Read the model definition and answer for the solid it produces. Units are mm, in the model's axes. A direction names the side the tool comes from. Give positions to 0.01 mm unless a question says otherwise; leave off trailing zeros. Order: outer loops, then holes, each group sorted by start corner. A loop starts at its lowest first (then second) coordinate and runs counter-clockwise, first axis right, second up.
Item 1: Given pin 1 Ø1.5 at (x, z) = (0.5, 5) entering from +Y; pin 2 Ø1.5 at (x, y) = (33.5, -19) entering from -Z; pin 3 Ø22.5 at (x, y) = (14, 0) entering from +Z; pin 4 Ø1.5 at (x, z) = (29, 19) entering from +Y, each flat-ended and moving along its own axis, determine where each tip first touches the part or whether it passes through.
Item 2: A cutting plane is placed at A-A (z = 10.25). Write down the section's boundary in (x, y).
Item 3: The mould has two halves that part along Y. Classify faces 4 (the face through (31.85, 19.07, 27.88)), 5 (the face through (23, 11, 0)), 6 (the face through (23.57, 10.22, 13.18)): +Y half, -Y half, draft (parallel to the pull), parting line (faces both ways), or undercut.
Item 4: Find the intervals of material crossed by line 1 along Z through (x, y) = (-7, 0.5); line 2 along Y through (x, z) = (25, 4.75); line 3 along X through (y, z) = (8, 4.5), in increasing order.
Item 5: Which of the six approach directions +Z, -Z, +X, -X, +Y, -Y give full straight-line access (tool end or side, diameter ignored) to faces 1 (the face through (14, -16, 19)), 2 (the face through (25, 12, 28)), 3 (the face through (27, 13, 25))?
from build123d import *

# Parameters (mm, degrees)
F1_ANGLE    = 270
F2_R        = 1.5
F3_T2_ANGLE = 300.5959645066
F4_R        = 2


# Not quite as in the source:
# - a fillet or chamfer that OpenCascade refuses, or shapes differently, is made with other operations: its cross-section is extruded or revolved along the edge and cut away or added


with BuildPart() as f1:
    # F0 (on Front) → F1 (revolve)
    with BuildSketch(Plane.XZ):
        Polygon((-2.5, 0), (0, 0), (0, 28), (-15, 28), (-15, 25), (-12.5, 25), (-2.5, 25), align=None)
    revolve(axis=Axis((14, 0, -3.1492561102), (0, 0, -1)), revolution_arc=F1_ANGLE)

    # F2
    f2_edges = [f1.edges().sort_by_distance(p)[0] for p in [
        (34.506097, 20.506097, 25),
    ]]
    fillet(f2_edges, radius=F2_R)

    # F3: chamfer of 3 on 1 edges, made by hand

    # F3_s1 → F3_t2 (revolve, cut)
    with BuildSketch(Plane(origin=(0.974554854, -3.562865531, 0), x_dir=(0, 0, 1), z_dir=(0.2638390816, -0.9645667105, 0))):
        Polygon((25, 15.496066053), (28, 12.496066053), (28, 15.496066053), align=None)
    revolve(axis=Axis((14, 0, 28), (0, 0, -1)), revolution_arc=F3_T2_ANGLE, mode=Mode.SUBTRACT)

    # F4
    f4_edges = [f1.edges().sort_by_distance(p)[0] for p in [
        (23.899495, 9.899495, 28),
    ]]
    fillet(f4_edges, radius=F4_R)


solid = f1.part
Response values:
1. pin 1: stops at y = 10.47
1. pin 2: stops at z = 25
1. pin 3: passes through
1. pin 4: stops at y = 8.32
2. outline: (-2.5, 0) - (0, 0) arc R14 cw (long way) to (14, -14) - (14, -16.5) arc R16.5 ccw (long way) to start
3. face 4: parting line
3. face 5: draft
3. face 6: undercut
4. line 1: z = 25 to 28
4. line 2: y = -12.3 to -8.66, 8.66 to 12.3
4. line 3: x = -0.43 to 2.51, 25.49 to 28.43
5. face 1: +Z, -Z, -X, -Y
5. face 2: +Z, +X, -X, +Y, -Y
5. face 3: -Z
